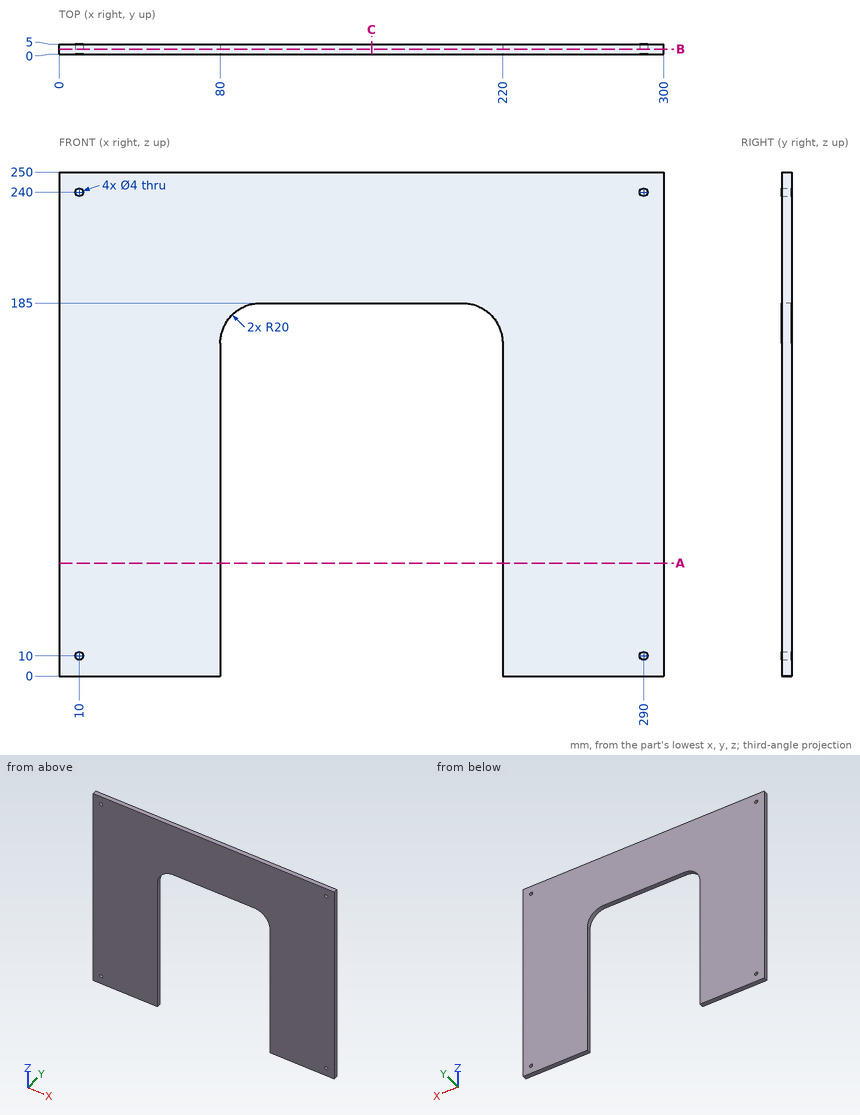
Design review of the part shown in the three views and the two pictorial views. Dimensions are in mm from the part's minimum x, y and z. Round coordinates to 2 decimals unless told otherwise and drop trailing zeros. Write each loop counter-clockwise with the first axis right and the second up, starting at its lowest first coordinate (ties: lowest second). Pieces come first, ordered by that corner, then holes. Notation, with made-up numbers: (35.25, 10.25) - (87.25, 10.25) arc R29 cw to (87.25, 39.25) - close; hole circle Ø10 at (21, -37.75). An arc over 180 degrees is marked (long way). Answer as CSV lines item,"result". Start each with the question number.
(1) Add section C-C, the plane x = 155. State the section outline as (y, z) points, plus the area to 3 significant figures.
(2) Add section B-B, the plane y = 2.45. State the section outline as (x, z) points.
(3) For line 1 (X direction, y = 3.7, z = 10); line 2 (Z direction, x = 290, y = 2.8); line 3 (X direction, y = 3.85, z = 99.5), list the stretches that pass through material, from the lowest coordinate up.
(4) For pin 1 (3 mm diameter, centred on x = 150.5, y = 3, fed in from -Z); pin 2 (3 mm diameter, centred on x = 290, z = 240, fed in from +Y), all flat-tipped, find the tip position at first contact; note any pin that passes through.
(5) Add section A-A, the plane z = 56. State the section outline as (x, y) points, plus the area to 3 significant figures.
From the geometry:
1,outline,"(0, 185) - (5, 185) - (5, 250) - (0, 250) - close"
1,area,"325 mm²"
2,outline,"(0, 0) - (80, 0) - (80, 165) arc R20 cw to (100, 185) - (200, 185) arc R20 cw to (220, 165) - (220, 0) - (300, 0) - (300, 250) - (0, 250) - close; hole circle Ø4 at (10, 10); hole circle Ø4 at (10, 240); hole circle Ø4 at (290, 10); hole circle Ø4 at (290, 240)"
3,line 1,"x = 0 to 8, 12 to 80, 220 to 288, 292 to 300"
3,line 2,"z = 0 to 8, 12 to 238, 242 to 250"
3,line 3,"x = 0 to 80, 220 to 300"
4,pin 1,"stops at z = 185"
4,pin 2,"passes through"
5,outline,"(0, 0) - (80, 0) - (80, 5) - (0, 5) - close; (220, 0) - (300, 0) - (300, 5) - (220, 5) - close"
5,area,"800 mm²"
